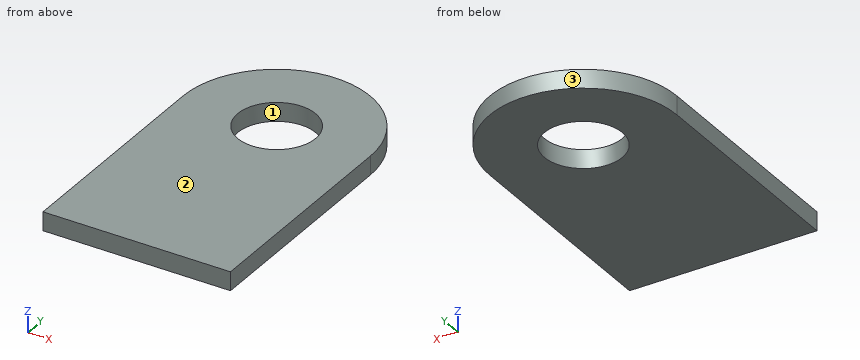
```python
from build123d import *

# Parameters (mm, degrees)
BOSS_EXTRUDE1_DEPTH  = 1.5875
M6_CLEARANCE_HOLE1_D = 6.6
SKETCH5_W            = 15.875
SKETCH5_H            = 6.35
CUT_EXTRUDE2_DEPTH   = 2.5875


with BuildPart() as part:
    # Sketch1 → Boss-Extrude1 (new body)
    with BuildSketch(Plane.XY):
        with BuildLine():
            Line((7.9375, -25.4), (7.9375, 0))
            ThreePointArc((7.9375, 0), (0, 7.9375), (-7.9375, 0))
            Line((-7.9375, 0), (-7.9375, -25.4))
            Line((-7.9375, -25.4), (7.9375, -25.4))
        make_face()
    extrude(amount=BOSS_EXTRUDE1_DEPTH)

    # M6 Clearance Hole1 (through all)
    with Locations(Plane.XY.offset(1.5875)):
        with Locations((0, 0)):
            Hole(M6_CLEARANCE_HOLE1_D / 2)

    # Sketch5 → Cut-Extrude2 (cut, through all)
    with BuildSketch(Plane.XY.offset(1.5875)):
        with Locations((0, -22.225)):
            Rectangle(SKETCH5_W, SKETCH5_H)
    extrude(amount=-CUT_EXTRUDE2_DEPTH, mode=Mode.SUBTRACT)


solid = part.part
```
Input: part model. Units: mm. Frame: model coordinates. Face numbers are marked on the shaded views. Give positions to 0.01 mm unless a question says otherwise; leave off trailing zeros. Order: outer loops, then holes, each group sorted by start corner. A loop starts at its lowest first (then second) coordinate and runs counter-clockwise, first axis right, second up.
1. Cut plane B-B (y = -2.25). Return loops of the section in (x, z).
Computed:
outline: (-7.94, 0) - (-2.41, 0) - (-2.41, 1.59) - (-7.94, 1.59) - close; (2.41, 0) - (7.94, 0) - (7.94, 1.59) - (2.41, 1.59) - close
2. Draft query along Y for the marked faces 1, 2 and 3. Return one class per face: released by +Y, released by -Y, zero draft, split by the parting line, or undercut.
Computed:
face 1: undercut
face 2: zero draft
face 3: released by +Y
3. Line query: probe 1 along Y at (x, z) = (0, 1.35); probe 2 along Y at (x, z) = (2.5, 0.65); probe 3 along Y at (x, z) = (5, 1.4). Output: solid intervals per line, ascending.
Computed:
probe 1: y = -19.05 to -3.3, 3.3 to 7.94
probe 2: y = -19.05 to -2.15, 2.15 to 7.53
probe 3: y = -19.05 to 6.16
4. Cut plane D-D (x = -4). Return loops of the section in (y, z), and give its area (3 significant figures).
Computed:
outline: (-19.05, 0) - (6.86, 0) - (6.86, 1.59) - (-19.05, 1.59) - close
area: 41.1 mm2
5. Pin query (flat end, axial travel): pin 1 Ø6 at (x, y) = (0, 0) entering from -Z. Return the tip coordinate at first contact, or that it passes through.
Computed:
pin 1: passes through
6. Cut plane A-A (x = 0). Return loops of the section in (y, z), and give its area (3 significant figures).
Computed:
outline: (-19.05, 0) - (-3.3, 0) - (-3.3, 1.59) - (-19.05, 1.59) - close; (3.3, 0) - (7.94, 0) - (7.94, 1.59) - (3.3, 1.59) - close
area: 32.4 mm2
